Input: part model. Units: mm. Frame: model coordinates. Face numbers are marked on the shaded views. A direction names the side the tool comes from. Coordinates: 2 decimals unless noted, no trailing zeros. Write each loop counter-clockwise with the first axis right and the second up, starting at its lowest first coordinate (ties: lowest second). Pieces come first, ordered by that corner, then holes. Notation, with made-up numbers: (11, -29.5) - (35, -29.5) arc R23 ccw to (35, 4.5) - close; hole circle Ø10 at (39, 45). An arc over 180 degrees is marked (long way). Use CSV: the item, a comma, the result in double quotes.
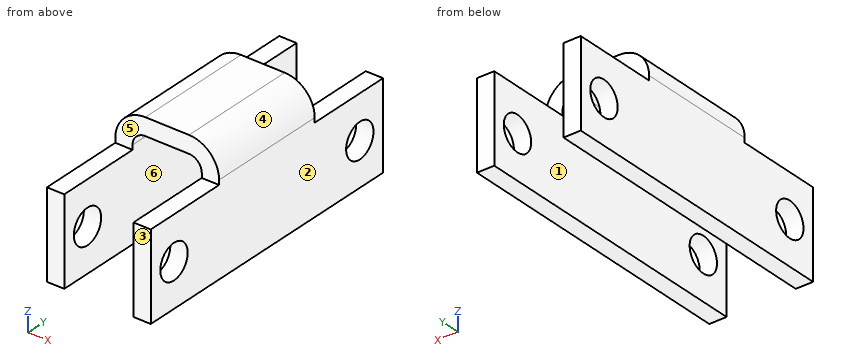
```python
from build123d import *

# Parameters (mm, degrees)
CROQUIS1_W                         = 6
CROQUIS1_H                         = 17
BRIDA_BASE1_DEPTH                  = 1
BRIDA_DE_ARISTA1_STRIP_W           = 5.4732
BRIDA_DE_ARISTA1_STRIP_H           = 1
BRIDA_DE_ARISTA1_STRIP_CUT_DEPTH   = 17
BRIDA_DE_ARISTA1_STRIP_2_W         = 5.4732
BRIDA_DE_ARISTA1_STRIP_2_H         = 1
BRIDA_DE_ARISTA1_STRIP_CUT_2_DEPTH = 17
BRIDA_DE_ARISTA1_DEPTH             = 17
BRIDA_DE_ARISTA1_BEND_DEPTH        = 17
CROQUIS12_W                        = 2
CROQUIS12_H                        = 5
CORTAR_EXTRUIR1_DEPTH              = 10
CROQUIS13_R                        = 1
CORTAR_EXTRUIR2_DEPTH              = 10


# Sheet-metal steps are written as plain solids
with BuildPart() as part:
    # Croquis1 → Brida base1 (new body)
    with BuildSketch(Plane.XY):
        with Locations((3, 8.5)):
            Rectangle(CROQUIS1_W, CROQUIS1_H)
    extrude(amount=-BRIDA_BASE1_DEPTH)

    # Brida de arista1 strip (across the edge) → Brida de arista1 strip cut (cut)
    with BuildSketch(Plane(origin=(6, 17, -1), x_dir=(-1, 0, 0), z_dir=(0, -1, 0))):
        with Locations((-1, -0.5)):
            Rectangle(BRIDA_DE_ARISTA1_STRIP_W, BRIDA_DE_ARISTA1_STRIP_H)
    extrude(amount=BRIDA_DE_ARISTA1_STRIP_CUT_DEPTH, mode=Mode.SUBTRACT)

    # Brida de arista1 strip 2 (across the edge) → Brida de arista1 strip cut 2 (cut)
    with BuildSketch(Plane(origin=(0, 0, -1), x_dir=(1, 0, 0), z_dir=(0, 1, 0))):
        with Locations((-1, -0.5)):
            Rectangle(BRIDA_DE_ARISTA1_STRIP_2_W, BRIDA_DE_ARISTA1_STRIP_2_H)
    extrude(amount=BRIDA_DE_ARISTA1_STRIP_CUT_2_DEPTH, mode=Mode.SUBTRACT)

    # Brida de arista1 section (across the edge) → Brida de arista1 (add)
    with BuildSketch(Plane(origin=(6, 17, -1), x_dir=(-1, 0, 0), z_dir=(0, -1, 0))):
        with BuildLine():
            Line((0, 0.7366), (0, 6))
            Line((0, 6), (1, 6))
            Line((1, 6), (1, 0.7366))
            ThreePointArc((1, 0.7366), (1.215745145, 0.215745145), (1.7366, 0))
            Line((1.7366, 0), (1.7366, -1))
            ThreePointArc((1.7366, -1), (0.508638364, -0.491361636), (0, 0.7366))
        make_face()
    extrude(amount=BRIDA_DE_ARISTA1_DEPTH)

    # Brida de arista1 section 2 (across the edge) → Brida de arista1 bend (add)
    with BuildSketch(Plane(origin=(0, 0, -1), x_dir=(1, 0, 0), z_dir=(0, 1, 0))):
        with BuildLine():
            Line((0, 0.7366), (0, 6))
            Line((0, 6), (1, 6))
            Line((1, 6), (1, 0.7366))
            ThreePointArc((1, 0.7366), (1.215745145, 0.215745145), (1.7366, 0))
            Line((1.7366, 0), (1.7366, -1))
            ThreePointArc((1.7366, -1), (0.508638364, -0.491361636), (0, 0.7366))
        make_face()
    extrude(amount=BRIDA_DE_ARISTA1_BEND_DEPTH)

    # Croquis12 → Cortar-Extruir1 (cut)
    with BuildSketch(Plane(origin=(6, 0, 0), x_dir=(0, 0, -1), z_dir=(1, 0, 0))):
        with Locations((1, 14.5)):
            Rectangle(CROQUIS12_W, CROQUIS12_H)
        with Locations((1, 2.5)):
            Rectangle(CROQUIS12_W, CROQUIS12_H)
    extrude(amount=-CORTAR_EXTRUIR1_DEPTH, mode=Mode.SUBTRACT)

    # Croquis13 → Cortar-Extruir2 (cut)
    with BuildSketch(Plane(origin=(6, 0, 0), x_dir=(0, 0, -1), z_dir=(1, 0, 0))):
        with Locations((4.5, 15.3)):
            Circle(CROQUIS13_R)
        with Locations((4.5, 1.7)):
            Circle(CROQUIS13_R)
    extrude(amount=-CORTAR_EXTRUIR2_DEPTH, mode=Mode.SUBTRACT)


solid = part.part
```
(1) Draft query along X for the marked faces 1, 2 and 3. Return one class per face: pulls with the +X half, pulls with the -X half, needs draft (parallel to the pull), parting line crosses it, or undercut.
Check values:
face 1,"undercut"
face 2,"pulls with the +X half"
face 3,"needs draft"
(2) Cut plane C-C on y = 15.3. Return loops of the section in (x, z), and give its area (3 significant figures).
Check values:
outline,"(0, -7) - (1, -7) - (1, -5.5) - (0, -5.5) - close; (0, -3.5) - (1, -3.5) - (1, -2) - (0, -2) - close; (5, -7) - (6, -7) - (6, -5.5) - (5, -5.5) - close; (5, -3.5) - (6, -3.5) - (6, -2) - (5, -2) - close"
area,"6.00 mm^2"
(3) Ray query, probe 1 along Y at (x, z) = (5.75, -4.5); probe 2 along X at (y, z) = (4.5, -5); probe 3 along Z at (x, y) = (5.35, 4.75). Return the intervals inside material, ascending. Write a range as from..to.
Check values:
probe 1,"0..0.7, 2.7..14.3, 16.3..17"
probe 2,"0..1, 5..6"
probe 3,"-7..-2"
(4) Cut plane B-B on z = -4.5. Return loops of the section in (x, y), and give its area (3 significant figures).
Check values:
outline,"(0, 0) - (1, 0) - (1, 0.7) - (0, 0.7) - close; (0, 2.7) - (1, 2.7) - (1, 14.3) - (0, 14.3) - close; (0, 16.3) - (1, 16.3) - (1, 17) - (0, 17) - close; (5, 0) - (6, 0) - (6, 0.7) - (5, 0.7) - close; (5, 2.7) - (6, 2.7) - (6, 14.3) - (5, 14.3) - close; (5, 16.3) - (6, 16.3) - (6, 17) - (5, 17) - close"
area,"26.0 mm^2"
(5) Cut plane D-D on z = -6. Return loops of the section in (x, y), and give its area (3 significant figures).
Check values:
outline,"(0, 0) - (1, 0) - (1, 17) - (0, 17) - close; (5, 0) - (6, 0) - (6, 17) - (5, 17) - close"
area,"34.0 mm^2"
(6) Pin query (flat end, axial travel): pin 1 Ø0.5 at (x, y) = (5.5, 14) entering from +Z; pin 2 Ø0.8 at (x, y) = (3, 10) entering from -Z; pin 3 Ø2 at (x, z) = (2.5, -1) entering from +Y. Return the tip coordinate at first contact, or that it passes through.
Check values:
pin 1,"z = -2"
pin 2,"z = -1"
pin 3,"y = 12"
(7) Cut plane A-A on y = 13. Return loops of the section in (x, z), and give its area (3 significant figures).
Check values:
outline,"(0, -7) - (1, -7) - (1, -2) - (0, -2) - close; (5, -7) - (6, -7) - (6, -2) - (5, -2) - close"
area,"10.0 mm^2"
(8) Reachability of the marked faces 4, 5 and 6 from +Z, -Z, +X, -X, +Y, -Y: full face, straight path, thin tool, end or side. Return the list, or none.
Check values:
face 4,"+Z, +X, +Y, -Y"
face 5,"+Z, +X, -X, -Y"
face 6,"-Z, +Y, -Y"
